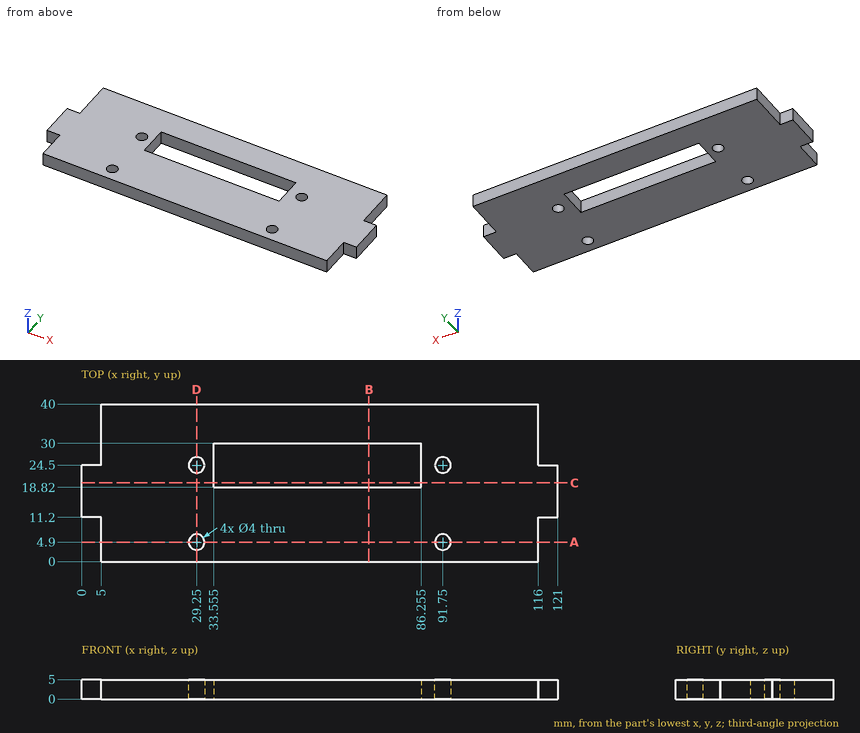
Answer from the drawing. Dimensions are ordinates in mm from the lowest x, y and z of the part. Round coordinates to 2 decimals unless told otherwise and drop trailing zeros. Write each loop counter-clockwise with the first axis right and the second up, starting at its lowest first coordinate (ties: lowest second). Pieces come first, ordered by that corner, then holes. Notation, with made-up numbers: (27, -9.75) - (59, -9.75) arc R29 ccw to (59, 21.25) - close; hole circle Ø10 at (45.25, -31.75). An arc over 180 degrees is marked (long way). One line per item, written item: value.
Q1. Each of these flat-tipped pins is pushed along its axis until it touches: P1, Ø1.5, axis at x = 119, z = 3, coming from the +Y side; P2, Ø1.5, axis at y = 26.5, z = 3.5, coming from the -X side; P3, Ø2.5, axis at x = 119, z = 2.5, coming from the -Y side; P4, Ø3.5, axis at x = 91.75, y = 4.9, coming from the -Z side. Where does it stop, or does it pass through?
The answers:
P1: stops at y = 24.5
P2: stops at x = 5
P3: stops at y = 11.2
P4: passes through
Q2. Find section D-D (x = 29.25). Determine the outline of the cut face in (y, z).
The answers:
outline: (0, 0) - (2.9, 0) - (2.9, 5) - (0, 5) - close; (6.9, 0) - (22.5, 0) - (22.5, 5) - (6.9, 5) - close; (26.5, 0) - (40, 0) - (40, 5) - (26.5, 5) - close
Q3. Straight lines are drawn through the part: line 1 (Y direction, x = 29.25, z = 1.3); line 2 (X direction, y = 28, z = 1.4) (1 decimal); line 3 (Y direction, x = 34, z = 1.55). For each, find the intervals that lie inside material, in ascending order. Write a range as from..to.
The answers:
line 1: y = 0..2.9, 6.9..22.5, 26.5..40
line 2: x = 5..33.6, 86.3..116
line 3: y = 0..18.82, 30..40
Q4. Find section A-A (y = 4.9). Determine the outline of the cut face in (x, z).
The answers:
outline: (5, 0) - (27.25, 0) - (27.25, 5) - (5, 5) - close; (31.25, 0) - (89.75, 0) - (89.75, 5) - (31.25, 5) - close; (93.75, 0) - (116, 0) - (116, 5) - (93.75, 5) - close
Q5. Find section C-C (y = 20). Determine the outline of the cut face in (x, z) (1 decimal).
The answers:
outline: (0, 0) - (33.6, 0) - (33.6, 5) - (0, 5) - close; (86.3, 0) - (121, 0) - (121, 5) - (86.3, 5) - close
Q6. Find section B-B (x = 73). Determine the outline of the cut face in (y, z).
The answers:
outline: (0, 0) - (18.82, 0) - (18.82, 5) - (0, 5) - close; (30, 0) - (40, 0) - (40, 5) - (30, 5) - close
